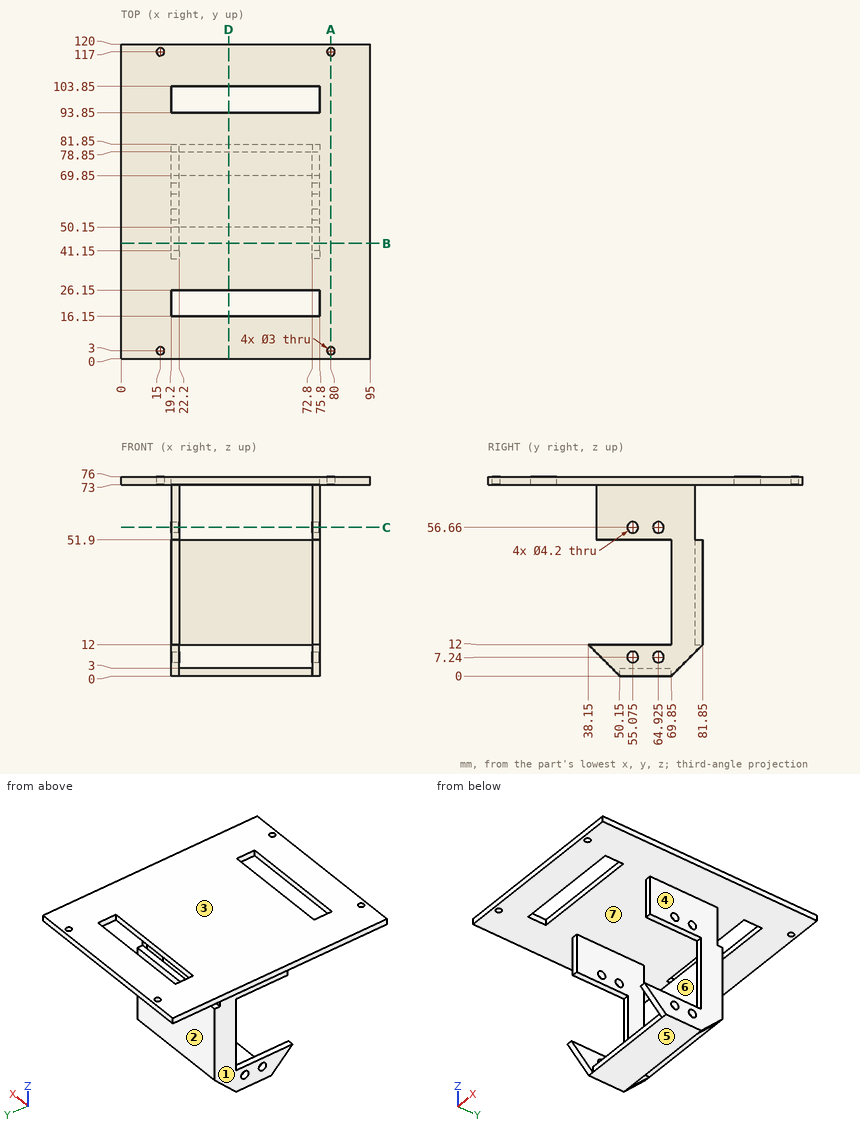
Input: dimensioned drawing with shaded views. Units: mm. Origin: part minimum x, y, z. A direction names the side the tool comes from. Round coordinates to 2 decimals unless told otherwise and drop trailing zeros. Order: outer loops, then holes, each group sorted by start corner. A loop starts at its lowest first (then second) coordinate and runs counter-clockwise, first axis right, second up. Notation, with made-up numbers: (-39, 82) - (10, 82) arc R14 ccw to (10, 109) - close; hole circle Ø8 at (29, -4.5). An arc over 180 degrees is marked (long way). Use CSV: the item, a comma, the result in double quotes. Start each with the question number.
Q1. Access query for the marked faces 1, 2 and 3. Directions: +Z, -Z, +X, -X, +Y, -Y. A direction counts if a zero-diameter tool reaches every point of the face in a straight line with its end or side. Return the directions, or none.
Q2. Section query A-A (x = 80). Return loops of the section in (y, z).
Q3. Section query C-C (z = 56.66). Return loops of the section in (x, y) (3 decimals), and give its area (3 significant figures).
Q4. Material intervals for line 1 along Y through (x, z) = (15, 73.85); line 2 along Y through (x, z) = (74.15, 56.66) (3 decimals); line 3 along Z through (x, y) = (40, 55.5), sorted ascending. Write a range as from..to.
Q5. Section query D-D (x = 41). Return loops of the section in (y, z), and give its area (3 significant figures).
Q6. Mould query, pull axis X, two halves, no side actions, for the marked faces 4, 5, 6 and 7. Classes: +X half, -X half, draft (parallel to the pull), parting line (faces both ways), or undercut.
Q7. First-contact query: pin 1 (1.5 mm diameter, centred on x = 54, z = 74.5, fed in from -Y); pin 2 (2 mm diameter, centred on x = 9.5, y = 104, fed in from -Z); pin 3 (2.5 mm diameter, centred on x = 20.5, z = 64.5, fed in from +Y); pin 4 (12 mm diameter, centred on x = 52.5, z = 18.5, fed in from -Y). Flat tips, straight axial feed; report the tip coordinate or a pass-through.
Q8. Section query B-B (y = 44). Return loops of the section in (x, z), and give its area (3 significant figures).
Result set:
1,face 1,"-Z, -X, +Y, -Y"
1,face 2,"-Z, +X, -X, +Y"
1,face 3,"+Z, +X, -X, +Y, -Y"
2,outline,"(0, 73) - (1.5, 73) - (1.5, 76) - (0, 76) - close; (4.5, 73) - (115.5, 73) - (115.5, 76) - (4.5, 76) - close; (118.5, 73) - (120, 73) - (120, 76) - (118.5, 76) - close"
3,outline,"(19.2, 41.15) - (22.2, 41.15) - (22.2, 52.975) - (19.2, 52.975) - close; (19.2, 57.175) - (22.2, 57.175) - (22.2, 62.825) - (19.2, 62.825) - close; (19.2, 67.025) - (22.2, 67.025) - (22.2, 78.85) - (19.2, 78.85) - close; (72.8, 41.15) - (75.8, 41.15) - (75.8, 52.975) - (72.8, 52.975) - close; (72.8, 57.175) - (75.8, 57.175) - (75.8, 62.825) - (72.8, 62.825) - close; (72.8, 67.025) - (75.8, 67.025) - (75.8, 78.85) - (72.8, 78.85) - close"
3,area,"176 mm2"
4,line 1,"y = 0..1.5, 4.5..115.5, 118.5..120"
4,line 2,"y = 41.15..52.975, 57.175..62.825, 67.025..78.85"
4,line 3,"z = 0..3, 73..76"
5,outline,"(0, 73) - (16.15, 73) - (16.15, 76) - (0, 76) - close; (26.15, 73) - (93.85, 73) - (93.85, 76) - (26.15, 76) - close; (50.15, 0) - (69.85, 0) - (69.85, 3) - (50.15, 3) - close; (78.85, 12) - (81.85, 12) - (81.85, 51.9) - (78.85, 51.9) - close; (103.85, 73) - (120, 73) - (120, 76) - (103.85, 76) - close"
5,area,"479 mm2"
6,face 4,"+X half"
6,face 5,"draft"
6,face 6,"undercut"
6,face 7,"undercut"
7,pin 1,"stops at y = 0"
7,pin 2,"stops at z = 73"
7,pin 3,"stops at y = 78.85"
7,pin 4,"stops at y = 78.85"
8,outline,"(0, 73) - (19.2, 73) - (19.2, 51.9) - (22.2, 51.9) - (22.2, 73) - (72.8, 73) - (72.8, 51.9) - (75.8, 51.9) - (75.8, 73) - (95, 73) - (95, 76) - (0, 76) - close; (19.2, 6.15) - (22.2, 6.15) - (22.2, 12) - (19.2, 12) - close; (72.8, 6.15) - (75.8, 6.15) - (75.8, 12) - (72.8, 12) - close"
8,area,"447 mm2"
